Could you check a few things on this drawing? It's one solid part, dimensions in mm from its lowest x, y, z. Give positions to 0.01 mm unless a question says otherwise; leave off trailing zeros. Order: outer loops, then holes, each group sorted by start corner. A loop starts at its lowest first (then second) coordinate and runs counter-clockwise, first axis right, second up. Notation, with made-up numbers: (11.5, -35.75) - (40.5, -35.75) arc R27 cw to (40.5, 1.25) - close; hole circle Ø7 at (15, -40). An arc over 180 degrees is marked (long way). Put each result on its own line as item: value.
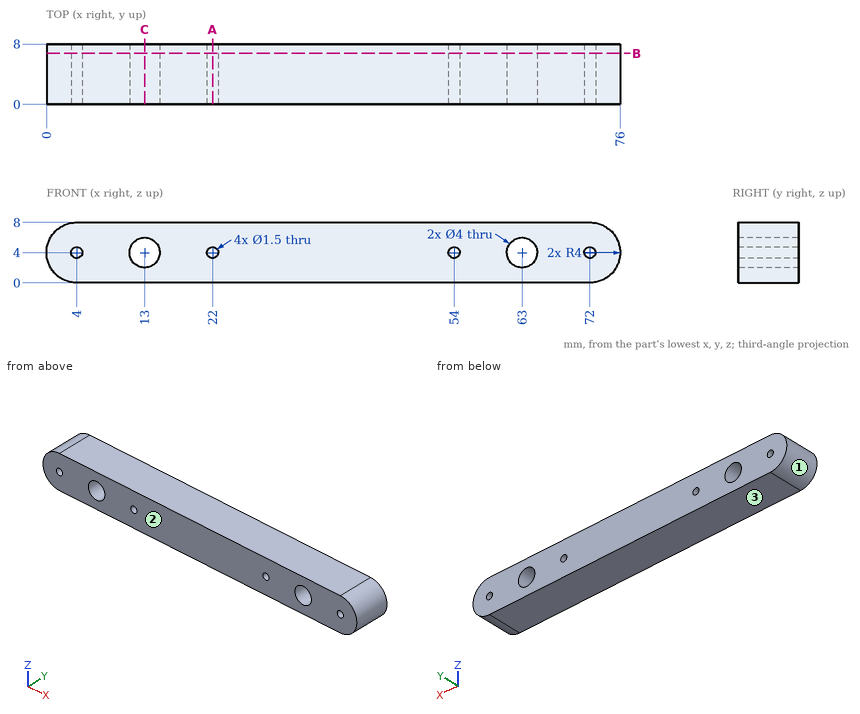
1) Suppose I cut it at B-B, the plane y = 6.75. List the corners of the cut face in (x, z) for me, and give its area (3 significant figures).
Filled in:
outline: (4, 0) - (72, 0) arc R4 ccw to (72, 8) - (4, 8) arc R4 ccw to start; hole circle Ø1.5 at (4, 4); hole circle Ø4 at (13, 4); hole circle Ø1.5 at (22, 4); hole circle Ø1.5 at (54, 4); hole circle Ø4 at (63, 4); hole circle Ø1.5 at (72, 4)
area: 562 mm^2
2) Suppose I cut it at A-A, the plane x = 22. List the corners of the cut face in (y, z) for me.
Filled in:
outline: (0, 0) - (8, 0) - (8, 3.25) - (0, 3.25) - close; (0, 4.75) - (8, 4.75) - (8, 8) - (0, 8) - close
3) Suppose I cut it at C-C, the plane x = 13. List the corners of the cut face in (y, z) for me, and give its area (3 significant figures).
Filled in:
outline: (0, 0) - (8, 0) - (8, 2) - (0, 2) - close; (0, 6) - (8, 6) - (8, 8) - (0, 8) - close
area: 32.0 mm^2
4) If I drill on line 1 (Z direction, x = 4, y = 2.25); line 2 (X direction, y = 4, z = 5.25); line 3 (Z direction, x = 14, y = 7.5), over which ranges is the centre line in solid material (lowest first)? Write a range as [from, to].
Filled in:
line 1: z = [0, 3.25], [4.75, 8]
line 2: x = [0.2, 11.44], [14.56, 61.44], [64.56, 75.8]
line 3: z = [0, 2.27], [5.73, 8]
5) We'd pull the mould along Z, two halves only. Please class the marked faces 1, 2 and 3: pulls with the +Z half, pulls with the -Z half, needs draft (parallel to the pull), parting line crosses it, or undercut.
Filled in:
face 1: parting line crosses it
face 2: needs draft
face 3: pulls with the -Z half
